The model under review builds one solid part; all positions refer to its coordinate system, in mm. Face numbers are marked on the shaded views. A direction names the side the tool comes from. Coordinates: 2 decimals unless noted, no trailing zeros. Order: outer loops, then holes, each group sorted by start corner. A loop starts at its lowest first (then second) coordinate and runs counter-clockwise, first axis right, second up. Notation, with made-up numbers: (-1.5, 26) -> (38.5, 26) arc R22 cw to (38.5, 63) -> close; hole circle Ø5 at (23, 86). An arc over 180 degrees is marked (long way). Use one line per item in the form item = value.
from build123d import *

# Parameters (mm, degrees)
F0_W      = 50
F0_H      = 50
F0_R      = 5
F1_DEPTH  = 16
F2_W      = 8
F2_H      = 2
F3_DEPTH  = 32.001
F4_R      = 3
F5_DEPTH  = 32.001
F6_R      = 4
F6_R_2    = 3
F7_DEPTH  = 24
F8_R      = 6
F9_DEPTH  = 18
F10_SIZE2 = 3
F10_SIZE  = 3
F12_D     = 2.5
F12_DEPTH = 8
F12_TIP   = 0.7510757738


with BuildPart() as f1:
    # F0 (on Top) → F1 (new body, symmetric)
    with BuildSketch(Plane.XY):
        Rectangle(F0_W, F0_H)
        Circle(F0_R, mode=Mode.SUBTRACT)
    extrude(amount=F1_DEPTH, both=True)

    # F2 (on face) → F3 (cut, through all)
    with BuildSketch(Plane.XY.offset(16)):
        with Locations((17, 24)):
            Rectangle(F2_W, F2_H)
    extrude(amount=-F3_DEPTH, mode=Mode.SUBTRACT)

    # F4 (on face) → F5 (cut, through all)
    with BuildSketch(Plane.XY.offset(16)):
        with Locations((5, 17)):
            Circle(F4_R)
    extrude(amount=-F5_DEPTH, mode=Mode.SUBTRACT)

    # F6 (on face) → F7 (cut)
    with BuildSketch(Plane.XY.offset(16)):
        with Locations((5, 17)):
            Circle(F6_R)
        with Locations((5, 17)):
            Circle(F6_R_2, mode=Mode.SUBTRACT)
    extrude(amount=-F7_DEPTH, mode=Mode.SUBTRACT)

    # F8 (on face) → F9 (cut)
    with BuildSketch(Plane(origin=(0, 25, 0), x_dir=(-1, 0, 0), z_dir=(0, 1, 0))):
        with Locations((-5, -1)):
            Circle(F8_R)
    extrude(amount=-F9_DEPTH, mode=Mode.SUBTRACT)

    # F10
    f10_edges = [f1.edges().sort_by_distance(p)[0] for p in [
        (2, 17, -16),
    ]]
    chamfer(f10_edges, length=F10_SIZE, length2=F10_SIZE2)

    # F12
    with Locations(Plane(origin=(0, 23, 0), x_dir=(-1, 0, 0), z_dir=(0, 1, 0))):
        with Locations((-17, 8), (-17, -8)):
            Hole(F12_D / 2, depth=F12_DEPTH)
            with Locations((0, 0, -(F12_DEPTH + F12_TIP / 2))):  # 118° drill point
                Cone(0, F12_D / 2, F12_TIP, mode=Mode.SUBTRACT)


solid = f1.part
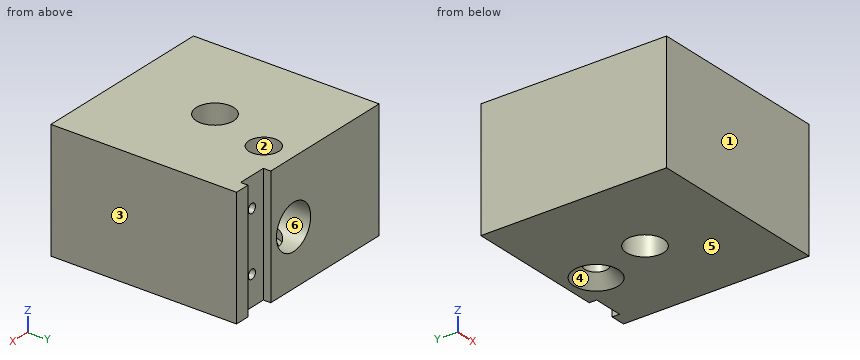
Item 1: To check wall thickness, follow L1, parallel to Z at x = 17, y = 18.75; L2, parallel to X at y = 17, z = 7; L3, parallel to Y at x = 17, z = -11. State the ranges of each line that lie inside material, in increasing order. Write a range as from..to.
Results found:
L1 = -16..-9.25, -6.75..6.75, 9.25..16
L2 = -25..1, 9..16.25, 17.75..25
L3 = -25..23
Item 2: We need section B-B (z = 12). Write out the cut boundary in (x, y), plus the area to 3 significant figures.
Results found:
outline = (-25, -25) -> (25, -25) -> (25, 25) -> (21, 25) -> (21, 23) -> (13, 23) -> (13, 25) -> (-25, 25) -> close; hole circle Ø10 at (0, 0); hole circle Ø8 at (5, 17)
area = 2,360 mm²
Item 3: We need section A-A (y = 17). Write out the cut boundary in (x, z), plus the area to 3 significant figures.
Results found:
outline = (-25, -16) -> (-1, -16) -> (2, -13) -> (2, -8) -> (1, -8) -> (1, -5.47) arc R6 cw to (1, 3.47) -> (1, 16) -> (-25, 16) -> close; (8, -13) -> (11, -16) -> (25, -16) -> (25, 16) -> (9, 16) -> (9, 3.47) arc R6 cw to (9, -5.47) -> (9, -8) -> (8, -8) -> close; hole circle Ø2.5 at (17, -8); hole circle Ø2.5 at (17, 8)
area = 1,320 mm²
Item 4: We need section C-C (y = 0). Write out the cut boundary in (x, z), plus the area to 3 significant figures.
Results found:
outline = (-25, -16) -> (-5, -16) -> (-5, 16) -> (-25, 16) -> close; (5, -16) -> (25, -16) -> (25, 16) -> (5, 16) -> close
area = 1,280 mm²
Item 5: Tool access review of the marked faces 5 and 6: name each direction out of +Z, -Z, +X, -X, +Y, -Y from which nothing blocks a thin tool from reaching the whole face with its end or side.
Results found:
face_5 = -Z, +X, -X, +Y, -Y
face_6 = +Y
Item 6: Draft analysis for pull direction Y (two halves, no side actions). For the marked faces 1, 2, 3 and 4, state which applies: released by +Y, released by -Y, zero draft, split by the parting line, or undercut.
Results found:
face_1 = released by -Y
face_2 = undercut
face_3 = zero draft
face_4 = undercut
Item 7: We need section D-D (z = -1). Write out the cut boundary in (x, y).
Results found:
outline = (-25, -25) -> (25, -25) -> (25, 25) -> (21, 25) -> (21, 23) -> (13, 23) -> (13, 25) -> (11, 25) -> (11, 7) -> (-1, 7) -> (-1, 25) -> (-25, 25) -> close; hole circle Ø10 at (0, 0)
Item 8: Clearance check with flat-ended pins moving along their axes: pin 1 (4 mm diameter, centred on x = 17, z = -8, fed in from +Y); pin 2 (9 mm diameter, centred on x = 5, y = 17, fed in from -Z); pin 3 (6 mm diameter, centred on x = 6, z = 0, fed in from +Y). State where each tip first meets the part, or that it passes through.
Results found:
pin_1 = 23
pin_2 = -14.5
pin_3 = 7
